Source: CAD feature listing. Evaluate the final solid. Frame: model axes, mm. Coordinates: 2 decimals unless noted, no trailing zeros. Write each loop counter-clockwise with the first axis right and the second up, starting at its lowest first coordinate (ties: lowest second). Pieces come first, ordered by that corner, then holes. Notation, with made-up numbers: (62.5, 11.25) - (87.5, 11.25) arc R19 ccw to (87.5, 43.25) - close; hole circle Ø4 at (-33.5, 66). An arc over 180 degrees is marked (long way). One line per item, written item: value.
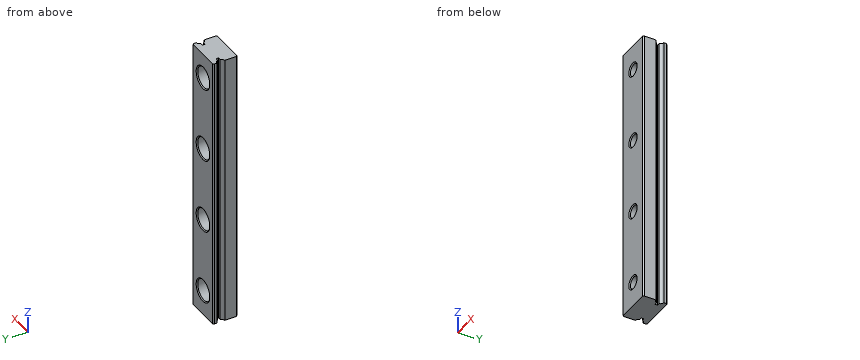
from build123d import *

# Parameters (mm, degrees)
EXTRUDE1_DEPTH             = 55
SKETCH2_R                  = 1.2
EXTRUDE2_DEPTH             = 4.8
SKETCH_R                   = 2.1
SKETCH_R_2                 = 1.2
EXTRUDE4_DEPTH             = 2.3
CHAMFER1_SIZE              = 0.2
LPATTERN1_COUNT            = 4
LPATTERN1_PITCH            = 15
CHAMFER1_OF_LPATTERN1_SIZE = 0.2


with BuildPart() as part:
    # Sketch1 → Extrude1 (new body)
    with BuildSketch(Plane.XY):
        with BuildLine():
            Line((-3.3, -2.4), (3.3, -2.4))
            Line((3.3, -2.4), (3.5, -2.2))
            Line((3.5, -2.2), (3.5, 0.106274607))
            ThreePointArc((3.5, 0.106274607), (3.091294745, 0.282570681), (2.840065792, 0.65))
            Line((2.840065792, 0.65), (2.340065792, 0.65))
            Line((2.340065792, 0.65), (2.340065792, 1.15))
            Line((2.340065792, 1.15), (2.840065792, 1.15))
            ThreePointArc((2.840065792, 1.15), (3.091294745, 1.517429319), (3.5, 1.693725393))
            Line((3.5, 1.693725393), (3.5, 2.2))
            Line((3.5, 2.2), (3.3, 2.4))
            Line((3.3, 2.4), (-3.3, 2.4))
            Line((-3.3, 2.4), (-3.5, 2.2))
            Line((-3.5, 2.2), (-3.5, 1.693725393))
            ThreePointArc((-3.5, 1.693725393), (-3.091294745, 1.517429319), (-2.840065792, 1.15))
            Line((-2.840065792, 1.15), (-2.340065792, 1.15))
            Line((-2.340065792, 1.15), (-2.340065792, 0.65))
            Line((-2.340065792, 0.65), (-2.840065792, 0.65))
            ThreePointArc((-2.840065792, 0.65), (-3.091294745, 0.282570681), (-3.5, 0.106274607))
            Line((-3.5, 0.106274607), (-3.5, -2.2))
            Line((-3.5, -2.2), (-3.3, -2.4))
        make_face()
    extrude(amount=EXTRUDE1_DEPTH)

    # Sketch2 → Extrude2 (cut)
    with BuildSketch(Plane(origin=(0, 2.4, 0), x_dir=(1, 0, 0), z_dir=(0, 1, 0))):
        with Locations((0, -5)):
            Circle(SKETCH2_R)
    extrude2 = extrude(amount=-EXTRUDE2_DEPTH, mode=Mode.SUBTRACT)

    # Sketch → Extrude4 (cut)
    with BuildSketch(Plane(origin=(0, 2.4, 0), x_dir=(1, 0, 0), z_dir=(0, 1, 0))):
        with Locations((0, -5)):
            Circle(SKETCH_R)
        with Locations((0, -5)):
            Circle(SKETCH_R_2, mode=Mode.SUBTRACT)
    extrude4 = extrude(amount=-EXTRUDE4_DEPTH, mode=Mode.SUBTRACT)

    # Chamfer1
    chamfer1_edges = [part.edges().sort_by_distance(p)[0] for p in [
        (-1.2, -2.4, 5),
        (-2.1, 2.4, 5),
    ]]
    chamfer(chamfer1_edges, length=CHAMFER1_SIZE)

    # LPattern1: Extrude2, Extrude4 ×4
    with Locations(*[(0, 0, i * LPATTERN1_PITCH) for i in range(1, LPATTERN1_COUNT)]):
        add(extrude2, mode=Mode.SUBTRACT)
        add(extrude4, mode=Mode.SUBTRACT)

    # Chamfer1 of LPattern1
    chamfer1_of_lpattern1_edges = [part.edges().sort_by_distance(p)[0] for p in [
        (-1.2, -2.4, 20),
        (-2.1, 2.4, 20),
        (-1.2, -2.4, 35),
        (-2.1, 2.4, 35),
        (-1.2, -2.4, 50),
        (-2.1, 2.4, 50),
    ]]
    chamfer(chamfer1_of_lpattern1_edges, length=CHAMFER1_OF_LPATTERN1_SIZE)


solid = part.part
1) Section query C-C on x = 0. State how many separate pieces and enclosed holes the cut face has, then the cut area to 3 significant figures.
Values found:
separate pieces: 5
enclosed holes: 0
area: 201 mm2
2) Contact query for flat-ended pins moving along their axis: P1, Ø4, axis at x = 0, z = 20, coming from the -Y side; P2, Ø2.5, axis at x = 0, z = 5, coming from the +Y side. Output: stop coordinate, or through.
Values found:
P1: y = -2.4
P2: y = 0.1
3) Material intervals for line 1 (Z direction, x = 0, y = -0.65); line 2 (Z direction, x = 0, y = 0.5); line 3 (X direction, y = 1, z = 5), sorted ascending.
Values found:
line 1: 0 to 3.8, 6.2 to 18.8, 21.2 to 33.8, 36.2 to 48.8, 51.2 to 55
line 2: 0 to 2.9, 7.1 to 17.9, 22.1 to 32.9, 37.1 to 47.9, 52.1 to 55
line 3: -2.34 to -2.1, 2.1 to 2.34
4) Section query A-A on y = -0.55. Output: boundary loops of the cut face in (x, z), then the cut area to 3 significant figures.
Values found:
outline: (-3.5, 0) - (3.5, 0) - (3.5, 55) - (-3.5, 55) - close; hole circle Ø2.4 at (0, 5); hole circle Ø2.4 at (0, 20); hole circle Ø2.4 at (0, 35); hole circle Ø2.4 at (0, 50)
area: 367 mm2
